Part model, mm, in its own coordinate system. A direction names the side the tool comes from. Give positions to 0.01 mm unless a question says otherwise; leave off trailing zeros. Write each loop counter-clockwise with the first axis right and the second up, starting at its lowest first coordinate (ties: lowest second). Pieces come first, ordered by that corner, then holes. Notation, with made-up numbers: (17, 75) - (54, 75) arc R5 ccw to (54, 80) - close; hole circle Ø6 at (80.5, -40). An arc over 180 degrees is marked (long way). Answer as a JSON object with one key per item and string values. Group by question number.
```python
from build123d import *

# Parameters (mm, degrees)
F2_W     = 120
F2_H     = 120
F3_DEPTH = 1680
F4_W     = 60
F4_H     = 80
F5_DEPTH = 120


with BuildPart() as f3:
    # F2 (on Top) → F3 (new body)
    with BuildSketch(Plane.XY):
        Rectangle(F2_W, F2_H)
    extrude(amount=F3_DEPTH)

    # F4 (on face) → F5 (cut, through all)
    with BuildSketch(Plane.XZ.offset(60)):
        with Locations((-30, 1640)):
            Rectangle(F4_W, F4_H)
    extrude(amount=-F5_DEPTH, mode=Mode.SUBTRACT)


solid = f3.part
```
1) Saw through at A-A (y = -38). List the corners of the cut face in (x, z).
2) Two-plate mould, pull along Z, no slides. Class faces 1 (the flat face through (-1, -60, 828)), 2 (the flat face through (-1, 1, 0)), 3 (the flat face through (30, 1, 1680)): +Z half, -Z half, draft (parallel to the pull), parting line (faces both ways), or undercut.
3) Drill centre line: line 1 along Z through (x, y) = (-53, -11.5). Where is it in solid material? Low to high. Write a range as from..to.
4) Drop a flat-ended pin along its axis: P1, Ø3, axis at x = -17.5, y = -36.5, coming from the +Z side. Give the stop position or say it passes through.
5) Which spindle directions (+Z, -Z, +X, -X, +Y, -Y) get a long thin tool onto all of the face, cutting with end or side? Do faces 4 (the flat face through (0, -1, 1639)), 5 (the flat face through (-1, 60, 828)). Say none if no direction does.
6) Saw through at B-B (x = -25). List the corners of the cut face in (y, z).
Checks:
{
 "1": {"outline": "(-60, 0) - (60, 0) - (60, 1680) - (0, 1680) - (0, 1600) - (-60, 1600) - close"},
 "2": {"face 1": "draft", "face 2": "-Z half", "face 3": "+Z half"},
 "3": {"line 1": "0..1600"},
 "4": {"P1": "z = 1600"},
 "5": {"face 4": "+Z, -X, +Y, -Y", "face 5": "+Z, -Z, +X, -X, +Y"},
 "6": {"outline": "(-60, 0) - (60, 0) - (60, 1600) - (-60, 1600) - close"}
}
